Read the model definition and answer for the solid it produces. Units are mm, in the model's axes. A direction names the side the tool comes from. Coordinates: 2 decimals unless noted, no trailing zeros. Loops run counter-clockwise (first coordinate to the right, second up) from the corner with the lowest first, then second, coordinate; pieces in that order, holes last. Notation, with made-up numbers: (81.5, 31.25) -> (92.5, 31.25) arc R11 cw to (92.5, 42.25) -> close; hole circle Ø6 at (-28.5, 65.25). An arc over 180 degrees is marked (long way). Answer as CSV lines item,"result".
```python
from build123d import *
from build123d import SkipClean  # not in build123d's __all__

# Parameters (mm, degrees)
F1_R     = 1.125
F1_R_2   = 1.5
F2_DEPTH = 3
F4_R     = 1
F4_W     = 7.5
F4_H     = 20
F5_DEPTH = 3
F6_R     = 1.5


with BuildPart() as f2:
    # F1 (on Front) → F2 (new body)
    with BuildSketch(Plane.XZ):
        with BuildLine():
            Line((0, 22), (0, 11))
            ThreePointArc((0, 11), (11, 0), (0, -11))
            Line((0, -11), (0, -33.375))
            ThreePointArc((0, -33.375), (2.1828294381, -33.3035415631), (4.3563116653, -33.0894722484))
            ThreePointArc((4.3563116653, -33.0894722484), (6.1795146274, -34.4884650857), (4.7805217901, -36.3116680478))
            ThreePointArc((4.7805217901, -36.3116680478), (2.3953896081, -36.5465830636), (0, -36.625))
            Line((0, -36.625), (0, -53))
            Line((0, -53), (14.5895357507, -53))
            Line((14.5895357507, -53), (21.3767935231, -78.330390851))
            Line((21.3767935231, -78.330390851), (29.104200163, -76.2598384823))
            Line((29.104200163, -76.2598384823), (21, -46.0145517191))
            Line((21, -46.0145517191), (21, 22))
            Line((21, 22), (0, 22))
        make_face()
        with Locations((21.3582111666, -62.8062272723)):
            Circle(F1_R, mode=Mode.SUBTRACT)
        with Locations((23.9464016176, -72.4654855352)):
            Circle(F1_R, mode=Mode.SUBTRACT)
        with Locations((15.5, -15.5)):
            Circle(F1_R_2, mode=Mode.SUBTRACT)
        with Locations((15.5, 15.5)):
            Circle(F1_R_2, mode=Mode.SUBTRACT)
    extrude(amount=F2_DEPTH)

    # F3: F2 across face


with BuildPart() as f2_1:
    add(f2.part, clean=False)
    with SkipClean():  # cleaning this boolean's faces spoils the solid; the shape is the same uncleaned
        add(f2.part.mirror(Plane(origin=(0, -1.5, -22.1875), x_dir=(0, -1, 0), z_dir=(-1, 0, 0))), clean=False)

    # F4 (on Front) → F5 (join)
    with BuildSketch(Plane.XZ):
        Polygon((38, 17), (38, 42), (30.5, 42), (30.5, 22), (21, 22), (21, 0), align=None)
        with Locations((34.75, 27)):
            Circle(F4_R, mode=Mode.SUBTRACT)
        with Locations((34.75, 37)):
            Circle(F4_R, mode=Mode.SUBTRACT)
        with Locations((-13.25, 32)):
            Rectangle(F4_W, F4_H)
        with Locations((-13.75, 27)):
            Circle(F4_R, mode=Mode.SUBTRACT)
        with Locations((-13.75, 37)):
            Circle(F4_R, mode=Mode.SUBTRACT)
    extrude(amount=F5_DEPTH)

    # F6
    f6_edges = [f2_1.edges().sort_by_distance(p)[0] for p in [
        (-21, -1.5, 22),
        (-17, -1.5, 42),
        (-9.5, -1.5, 42),
        (30.5, -1.5, 42),
        (38, -1.5, 42),
        (38, -1.5, 17),
        (21, -1.5, 0),
        (21, -1.5, -46.014552),
        (29.1042, -1.5, -76.259838),
        (21.376794, -1.5, -78.330391),
        (-14.589536, -1.5, -53),
        (-21.376794, -1.5, -78.330391),
        (-29.1042, -1.5, -76.259838),
        (14.589536, -1.5, -53),
        (-21, -1.5, -46.014552),
        (-17, -1.5, 22),
    ]]
    fillet(f6_edges, radius=F6_R)


solid = f2_1.part
```
Q1. A cutting plane is placed at B-B, the plane z = -35. Write down the section's boundary in (x, y).
Results:
outline,"(-21, -3) -> (-6.17, -3) -> (-6.17, 0) -> (-21, 0) -> close; (6.17, -3) -> (21, -3) -> (21, 0) -> (6.17, 0) -> close"
Q2. Given pin 1 Ø2.5 at (x, z) = (-15.5, -15.5) entering from +Y; pin 2 Ø1.5 at (x, y) = (7.5, -1) entering from +Z; pin 3 Ø1 at (y, z) = (-1.5, -13.5) entering from -X; pin 4 Ø0.9 at (y, z) = (-1.5, 31) entering from -X, each flat-ended and moving along its own axis, determine where each tip first touches the part or whether it passes through.
Results:
pin 1,"passes through"
pin 2,"stops at z = 22"
pin 3,"stops at x = -21"
pin 4,"stops at x = -17"
Q3. A cutting plane is placed at C-C, the plane y = -0.45. Give the number of separate pieces and of enclosed holes in the cut face, and give its area (3 significant figures).
Results:
separate pieces,"1"
enclosed holes,"14"
area,"3,620 mm²"
Q4. For faces 1 (the face through (29, -1, 8)), 2 (the face through (17.895, -1.479, -65.337)), 3 (the face through (11, -1, 22)), determine the directions among +Z, -Z, +X, -X, +Y, -Y from which every point of the face is accessible in a straight line to the end or side of a thin tool.
Results:
face 1,"+X, +Y, -Y"
face 2,"-Z, +Y, -Y"
face 3,"+Z, +Y, -Y"
Q5. Find the intervals of material crossed by probe 1 along X at (y, z) = (-0.6, -63.5); probe 2 along X at (y, z) = (-0.1, 31.5); probe 3 along Z at (x, y) = (-13.75, -1.2), in increasing order. Write a range as [from, to].
Results:
probe 1,"x = [-25.69, -22.24], [-20.47, -17.4], [17.4, 20.47], [22.24, 25.69]"
probe 2,"x = [-17, -9.5], [30.5, 38]"
probe 3,"z = [-53.03, 26], [28, 36], [38, 42]"
Q6. A cutting plane is placed at A-A, the plane z = 30. Write down the section's boundary in (x, y).
Results:
outline,"(-17, -3) -> (-9.5, -3) -> (-9.5, 0) -> (-17, 0) -> close; (30.5, -3) -> (38, -3) -> (38, 0) -> (30.5, 0) -> close"
